Read the model definition and answer for the solid it produces. Units are mm, in the model's axes. Face numbers are marked on the shaded views. A direction names the side the tool comes from. Coordinates: 2 decimals unless noted, no trailing zeros. Order: outer loops, then holes, each group sorted by start corner. A loop starts at its lowest first (then second) coordinate and runs counter-clockwise, first axis right, second up. Notation, with made-up numbers: (40.25, 89) -> (62.25, 89) arc R15 ccw to (62.25, 106) -> close; hole circle Ø10 at (-15.75, 39). An arc over 180 degrees is marked (long way). Answer as a JSON object with one key per item and string values. Group by question number.
1) Section C-C on x = -21.5 is taken. Count the separate pieces of the cut face and the enclosed holes in it, and give its area (3 significant figures).
2) Section D-D on z = 130 is taken. Determine the outline of the cut face in (x, y), and give its area (3 significant figures).
3) Consider L1, parallel to Y at x = 0, z = 56; L2, parallel to Y at x = -1, z = 159; L3, parallel to Z at x = 1, y = 45.5. Determine where each line is inside the solid, lowest interval first.
4) A tool of negligible diameter and unlimited length cuts with its end or side. For the marked faces 1, 2 and 3, from which of +Z, -Z, +X, -X, +Y, -Y can it reach the whole face along a straight path? Write none if from no direction.
5) Determine the mould class of the marked faces 4, 5 and 6 for opening direction Y: released by +Y, released by -Y, zero draft, split by the parting line, or undercut.
6) Section B-B on z = 100 is taken. Determine the outline of the cut face in (x, y), and give its area (3 significant figures).
7) Given pin 1 (1.5 mm diameter, centred on x = -5, z = 60, fed in from -Y); pin 2 (3 mm diameter, centred on x = 13.5, y = 44.5, fed in from +Z); pin 3 (6 mm diameter, centred on y = -20.5, z = 143.5, fed in from +X); pin 4 (3 mm diameter, centred on x = -23.5, y = 8.5, fed in from -Z), each flat-ended and moving along its own axis, determine where each tip first touches the part or whether it passes through.
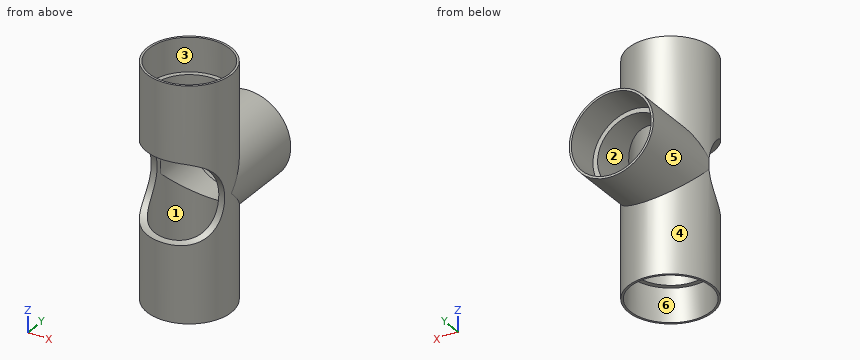
Autodesk Inventor part; units mm, degrees
ref_plane "Work Plane5" through (0, 31.75, 174.625) normal (0, 1, 0) x (-1, 0, 0)
ref_plane "Work Plane9" through (-31.2676, 5.5133, 174.625) normal (-0.9848, 0.1736, 0) x (-0.1736, -0.9848, 0)
ref_plane "YZ Plane" through (0, 0, 0) normal (1, 0, 0) x (0, 1, 0)
sketch "Sketch1" plane through (0, 0, 0) normal (0, 0, 1) x (1, 0, 0)
  circle A0 centre (0, 0) radius 31.75
  dimension "d0" = 63.5
extrude "mainBody" add sketch "Sketch1" along normal blind 174.625
sketch "Sketch10" plane through (0, 0, 174.625) normal (0, 0, 1) x (1, 0, 0)
  circle A0 centre (0, 0) radius 30.1625
  circle A1 centre (0, 0) radius 31.75
  point P0 (0, 31.75)
ref_plane "Work Plane5" through (0, 31.75, 174.625) normal (0, 1, 0) x (-1, 0, 0)
sketch "Sketch11" plane through (0, 31.75, 174.625) normal (0, 1, 0) x (-1, 0, 0)
  circle A0 centre (0, -87.3125) radius 31.75
  line L0 (31.75, 0) -> (-31.75, 0)
  point P0 (0, -174.625)
  dimension "d29" = 87.3125
  dimension "d30" = 63.5
extrude "TBody" add sketch "Sketch11" along normal blind 38.1 and the other way blind 31.75
sketch "Sketch12" plane through (0, 69.85, 87.3125) normal (0, 1, 0) x (1, 0, 0)
  circle A0 centre (0, 0) radius 31.75
  circle A1 centre (0, 0) radius 30.1625
  point P0 (0, 87.3125)
  dimension "d35" = 60.325
extrude "TSocket" cut sketch "Sketch12" against normal blind 25.4 contours A1
sketch "Sketch13" plane through (0, 44.45, 87.3125) normal (0, 1, 0) x (1, 0, 0)
  circle A0 centre (0, 0) radius 30.1625
  circle A1 centre (0, 0) radius 26.67
  point P0 (0, 87.3125)
  dimension "d39" = 53.34
extrude "TTube" cut sketch "Sketch13" against normal blind 38.1 contours A1
sketch "Sketch14" plane through (0, 0, 174.625) normal (0, 0, 1) x (1, 0, 0)
  circle A0 centre (0, 0) radius 31.75
  circle A1 centre (0, 0) radius 26.67
  dimension "d43" = 53.34
extrude "mainTube" cut sketch "Sketch14" against normal blind 177.8 contours A1
sketch "Sketch15" plane through (0, 0, 174.625) normal (0, 0, 1) x (1, 0, 0)
  circle A0 centre (0, 0) radius 26.67
  circle A1 centre (0, 0) radius 31.75
  circle A2 centre (0, 0) radius 30.1625
  dimension "d47" = 60.325
extrude "mainSocket1" cut sketch "Sketch15" against normal blind 25.4 contours A2
sketch "Sketch16" plane through (0, 0, 0) normal (0, 0, -1) x (-1, 0, 0)
  circle A0 centre (0, 0) radius 26.67
  circle A1 centre (0, 0) radius 31.75
  circle A2 centre (0, 0) radius 30.1625
  dimension "d51" = 60.325
extrude "mainSocket2" cut sketch "Sketch16" against normal blind 25.4 contours A2
sketch "Sketch23" plane through (0, 0, 174.625) normal (0, 0, 1) x (1, 0, 0)
  circle A0 centre (0, 0) radius 30.1625
  circle A1 centre (0, 0) radius 31.75
  line L0 (0, 0) -> (-50.0282, 8.8213)
  line L1 (0, 0) -> (50.8, 0) construction
  line L2 (-55.321, -21.1956) -> (-2.6667, -30.48)
  line L3 (-2.6667, -30.48) -> (50.8, -30.48)
  line L4 (-29.3824, 16.2053) -> (-36.5604, -24.5036)
  point P0 (-31.2676, 5.5133)
  dimension "d67" = 50.8
  dimension "d68" = 170
  dimension "d69" = 30.48
ref_plane "Work Plane9" through (-31.2676, 5.5133, 174.625) normal (-0.9848, 0.1736, 0) x (-0.1736, -0.9848, 0)
sketch "Sketch24" plane through (-31.2676, 5.5133, 174.625) normal (-0.9848, 0.1736, 0) x (-0.1736, -0.9848, 0)
  circle A0 centre (31.75, -87.3125) radius 30.48
  point P0 (0, -174.625)
  dimension "d70" = 60.96
extrude "Extrusion18" cut sketch "Sketch24" along normal mid plane 203.2
properties part number "pvc_tee" material "PVC-Piping"
Worked answers:
{
 "1": {"separate pieces": "4", "enclosed holes": "0", "area": "1,850 mm²"},
 "2": {"outline": "circle Ø63.5 at (0, 0); hole circle Ø53.34 at (0, 0)", "area": "932 mm²"},
 "3": {"L1": "y = -31.75 to -26.67, 26.67 to 69.85", "L2": "y = -31.73 to -30.15, 30.15 to 31.73", "L3": "z = 55.58 to 57.17, 117.46 to 119.05"},
 "4": {"face 1": "+Z, -Z", "face 2": "+Y", "face 3": "+Z"},
 "5": {"face 4": "split by the parting line", "face 5": "zero draft", "face 6": "undercut"},
 "6": {"outline": "(-31.71, 1.49) -> (-26.66, 0.6) arc R26.67 cw to (-23.46, 12.69) -> (-23.46, 44.45) -> (-27.36, 44.45) -> (-27.36, 69.85) -> (-29.1, 69.85) -> (-29.1, 12.69) arc R31.75 ccw to start; (23.46, 12.69) arc R26.67 cw to (25.26, -8.55) -> (30.31, -9.44) arc R31.75 ccw to (29.1, 12.69) -> (29.1, 69.85) -> (27.36, 69.85) -> (27.36, 44.45) -> (23.46, 44.45) -> close", "area": "622 mm²"},
 "7": {"pin 1": "stops at y = 26.04", "pin 2": "stops at z = 116.71", "pin 3": "stops at x = 26.49", "pin 4": "passes through"}
}
